CAD build for the part. Positions are in the model's coordinates, mm. Face numbers are marked on the shaded views. Coordinates: 2 decimals unless noted, no trailing zeros. Order: outer loops, then holes, each group sorted by start corner. A loop starts at its lowest first (then second) coordinate and runs counter-clockwise, first axis right, second up. Notation, with made-up numbers: M -3,89 L 11,89 A13 cw 11,113 Z; hole C 39.25,-25.5 d10. An arc over 180 degrees is marked long. Write item = value, one per line.
from build123d import *

# Parameters (mm, degrees)
SKETCH1_R           = 57.5
SKETCH1_R_2         = 52.5
BOSS_EXTRUDE1_DEPTH = 10
SKETCH2_R           = 1.45
BOSS_EXTRUDE2_DEPTH = 90
SKETCH4_R           = 57.227664134
BOSS_EXTRUDE3_DEPTH = 5


with BuildPart() as part:
    # Sketch1 → Boss-Extrude1 (new body)
    with BuildSketch(Plane(origin=(0, 0, 0), x_dir=(1, 0, 0), z_dir=(0, 1, 0))):
        Circle(SKETCH1_R)
        Circle(SKETCH1_R_2, mode=Mode.SUBTRACT)
    extrude(amount=BOSS_EXTRUDE1_DEPTH)

    # Sketch2 → Boss-Extrude2 (add)
    with BuildSketch(Plane.XZ):
        with Locations((0, 55)):
            Circle(SKETCH2_R)
        with Locations((1.578223765, -55)):
            Circle(SKETCH2_R)
        with Locations((55, 0)):
            Circle(SKETCH2_R)
        with Locations((-55, -1.760313132)):
            Circle(SKETCH2_R)
    extrude(amount=BOSS_EXTRUDE2_DEPTH)

    # Sketch4 → Boss-Extrude3 (add)
    with BuildSketch(Plane(origin=(0, -90, 0), x_dir=(-1, 0, 0), z_dir=(0, -1, 0))):
        Circle(SKETCH4_R)
    extrude(amount=BOSS_EXTRUDE3_DEPTH)


solid = part.part
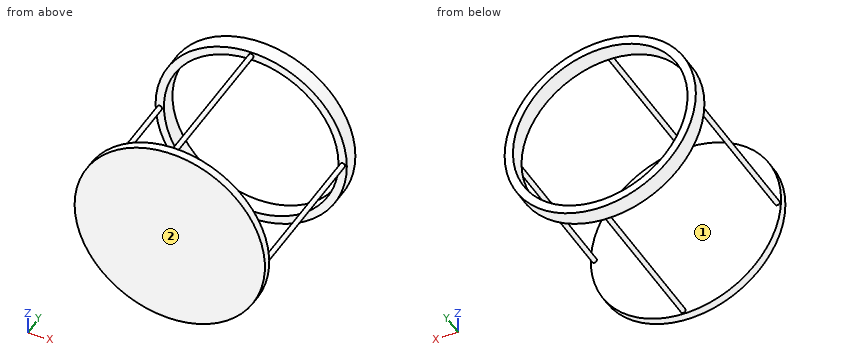
(1) Slice it at C-C, the plane y = -71.5. Write the cut outline in (x, z), then the cut area to 3 significant figures.
Evaluation:
outline = C -55,-1.76 d2.9; C 0,55 d2.9; C 1.58,-55 d2.9; C 55,0 d2.9
area = 26.4 mm²
(2) Pull direction Y, two halves, no side cores. Call the marked faces 1 and 2: +Y half, -Y half, draft (parallel to the pull), parting line (faces both ways), or undercut.
Evaluation:
face_1 = undercut
face_2 = -Y half
(3) Slice it at A-A, the plane x = -41. Write the cut outline in (y, z) (3 decimals), then the cut area to 3 significant figures.
Evaluation:
outline = M -95,-39.925 L -90,-39.925 L -90,39.925 L -95,39.925 Z; M 0,-40.314 L 10,-40.314 L 10,-32.791 L 0,-32.791 Z; M 0,32.791 L 10,32.791 L 10,40.314 L 0,40.314 Z
area = 550 mm²
(4) Slice it at B-B, the plane z = 15. Write the cut outline in (x, y), then the cut area to 3 significant figures.
Evaluation:
outline = M -55.51,0 L -50.31,0 L -50.31,10 L -55.51,10 Z; M -55.23,-95 L 55.23,-95 L 55.23,-90 L -55.23,-90 Z; M 50.31,0 L 55.51,0 L 55.51,10 L 50.31,10 Z
area = 656 mm²
(5) Wall check: line 1 (X direction, y = 5, z = 0); line 2 (Y direction, x = -41, z = -38.5). Give the ranges that are in metal, low to high. Write a range as from..to.
Evaluation:
line_1 = -57.5..-52.5, 52.5..57.5
line_2 = -95..-90, 0..10
(6) Pin check, flat tips, straight feed: pin 1 Ø2 at (y, z) = (-52, -3.5) entering from -X; pin 2 Ø2 at (y, z) = (-40, -4) entering from -X; pin 3 Ø2 at (x, z) = (39, 43.5) entering from -Y. Stop position of each tip, or through.
Evaluation:
pin_1 = -56.25
pin_2 = -55.75
pin_3 = 0
